```python
from build123d import *

# Parameters (mm, degrees)
SKETCH1_W           = 32.3215
SKETCH1_H           = 21.1455
SKETCH1_W_2         = 28.33878
SKETCH1_H_2         = 17.16278
BOSS_EXTRUDE1_DEPTH = 7.9375
SKETCH2_R           = 3.175
CUT_EXTRUDE1_DEPTH  = 37.1475
SKETCH3_R           = 3.302
CUT_EXTRUDE2_DEPTH  = 20.32
SKETCH4_R           = 1.778
BOSS_EXTRUDE3_DEPTH = 5.08
SKETCH6_R           = 0.9144
CUT_EXTRUDE3_DEPTH  = 10.922


with BuildPart() as part:
    # Sketch1 → Boss-Extrude1 (new body)
    with BuildSketch(Plane(origin=(0, 0, 0), x_dir=(1, 0, 0), z_dir=(0, 1, 0))):
        Rectangle(SKETCH1_W, SKETCH1_H)
        Rectangle(SKETCH1_W_2, SKETCH1_H_2, mode=Mode.SUBTRACT)
    extrude(amount=BOSS_EXTRUDE1_DEPTH)

    # Sketch2 → Cut-Extrude1 (cut)
    with BuildSketch(Plane.ZY.offset(16.16075)):
        with Locations((0, 3.96875)):
            Circle(SKETCH2_R)
    extrude(amount=-CUT_EXTRUDE1_DEPTH, mode=Mode.SUBTRACT)

    # Sketch3 → Cut-Extrude2 (cut)
    with BuildSketch(Plane.XY.offset(10.57275)):
        with Locations((0, 3.96875)):
            Circle(SKETCH3_R)
    extrude(amount=-CUT_EXTRUDE2_DEPTH, mode=Mode.SUBTRACT)

    # Sketch4 → Boss-Extrude3 (add)
    with BuildSketch(Plane(origin=(0, 0, -10.57275), x_dir=(-1, 0, 0), z_dir=(0, 0, -1))):
        with Locations(Location((0, 3.96875, 0), (0, 0, 180))):
            Circle(SKETCH4_R)
    extrude(amount=BOSS_EXTRUDE3_DEPTH)

    # Sketch6 → Cut-Extrude3 (cut)
    with BuildSketch(Plane(origin=(0, 0, -15.65275), x_dir=(-1, 0, 0), z_dir=(0, 0, -1))):
        with Locations((0, 3.96875)):
            Circle(SKETCH6_R)
    extrude(amount=-CUT_EXTRUDE3_DEPTH, mode=Mode.SUBTRACT)


solid = part.part
```
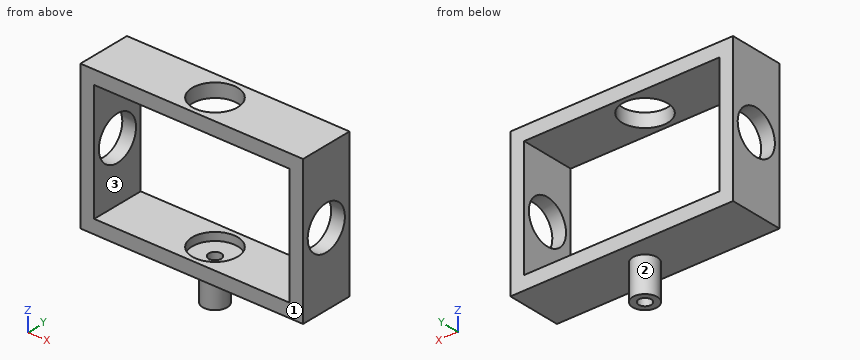
Work out the finished part from the listing and answer in its coordinate system (mm). Face numbers are marked on the shaded views. A direction names the side the tool comes from. Round coordinates to 2 decimals unless told otherwise and drop trailing zeros. Order: outer loops, then holes, each group sorted by start corner. A loop starts at its lowest first (then second) coordinate and runs counter-clockwise, first axis right, second up.
Q1. A cutting plane is placed at D-D, the plane x = 0. Determine the outline of the cut face in (y, z), then the cut area to 3 significant figures.
Solution:
outline: (0, -10.57) - (2.19, -10.57) - (2.19, -15.65) - (3.05, -15.65) - (3.05, -9.75) - (0.67, -9.75) - (0.67, -8.58) - (0, -8.58) - close; (0, 8.58) - (0.67, 8.58) - (0.67, 10.57) - (0, 10.57) - close; (4.88, -15.65) - (5.75, -15.65) - (5.75, -10.57) - (7.94, -10.57) - (7.94, -8.58) - (7.27, -8.58) - (7.27, -9.75) - (4.88, -9.75) - close; (7.27, 8.58) - (7.94, 8.58) - (7.94, 10.57) - (7.27, 10.57) - close
area: 18.0 mm2
Q2. A cutting plane is placed at B-B, the plane z = 0. Determine the outline of the cut face in (x, y).
Solution:
outline: (-16.16, 0) - (-14.17, 0) - (-14.17, 0.79) - (-16.16, 0.79) - close; (-16.16, 7.14) - (-14.17, 7.14) - (-14.17, 7.94) - (-16.16, 7.94) - close; (14.17, 0) - (16.16, 0) - (16.16, 0.79) - (14.17, 0.79) - close; (14.17, 7.14) - (16.16, 7.14) - (16.16, 7.94) - (14.17, 7.94) - close
Q3. A cutting plane is placed at C-C, the plane z = 6.25. Determine the outline of the cut face in (x, y), then the cut area to 3 significant figures.
Solution:
outline: (-16.16, 0) - (-14.17, 0) - (-14.17, 7.94) - (-16.16, 7.94) - close; (14.17, 0) - (16.16, 0) - (16.16, 7.94) - (14.17, 7.94) - close
area: 31.6 mm2
Q4. A cutting plane is placed at A-A, the plane x = 12. Determine the outline of the cut face in (y, z).
Solution:
outline: (0, -10.57) - (7.94, -10.57) - (7.94, -8.58) - (0, -8.58) - close; (0, 8.58) - (7.94, 8.58) - (7.94, 10.57) - (0, 10.57) - close
Q5. Find the intervals of material crossed by line 1 along Y through (x, z) = (0, -11.95); line 2 along Y through (x, z) = (0, -9.3); line 3 along Z through (x, y) = (5.5, 5.25), in increasing order.
Solution:
line 1: y = 2.19 to 3.05, 4.88 to 5.75
line 2: y = 0 to 0.67, 7.27 to 7.94
line 3: z = -10.57 to -8.58, 8.58 to 10.57
Q6. Given pin 1 Ø4 at (x, y) = (0, 3.97) entering from +Z; pin 2 Ø2.5 at (y, z) = (3, 1.5) entering from -X, each flat-ended and moving along its own axis, determine where each tip first touches the part or whether it passes through.
Solution:
pin 1: stops at z = -9.75
pin 2: passes through
Q7. A tool of negligible diameter and unlimited length cuts with its end or side. For the marked faces 1, 2 and 3, from which of +Z, -Z, +X, -X, +Y, -Y can it reach the whole face along a straight path? Write none if from no direction.
Solution:
face 1: +Z, -Z, +X, -X, -Y
face 2: -Z
face 3: +Y, -Y
